from build123d import *

# Parameters (mm, degrees)
BOSS_EXTRUDE1_DEPTH     = 19.05
BOSS_EXTRUDE2_DEPTH     = 19.05
FILLET1_R               = 3.175
FILLET2_R               = 12.7
CUT_EXTRUDE1_DEPTH      = 957.630297054
CUT_EXTRUDE1_DEPTH_BACK = 957.630297054
SKETCH47_R              = 3.175
FILLET4_R               = 6.35
F_0_25_DIAMETER_HOLE1_D = 6.35
HOLE6_D                 = 3.175
HOLE6_DEPTH             = 38.1
HOLE6_CSINK_D           = 10.16
HOLE6_CSINK_ANGLE       = 82
HOLE6_TIP               = 0.953866233
HOLE9_D                 = 3.175
HOLE9_DEPTH             = 57.15
HOLE9_CSINK_D           = 10.16
HOLE9_CSINK_ANGLE       = 82
HOLE9_TIP               = 0.953866233
HOLE15_D                = 3.175
HOLE15_DEPTH            = 31.75
HOLE15_CSINK_D          = 10.16
HOLE15_CSINK_ANGLE      = 82
HOLE15_TIP              = 0.953866233


with BuildPart() as part:
    # Sketch1 → Boss-Extrude1 (new body)
    with BuildSketch(Plane.XY):
        Polygon((-247.274665566, 82.142339986), (-313.471036221, 60.427634584), (-546.587167873, 771.072405964), (-504.525442447, 784.870110692), (-417.251419261, 518.818903446), (-393.116774032, 526.735904121), align=None)
    extrude(amount=-BOSS_EXTRUDE1_DEPTH)

    # Sketch2 → Boss-Extrude2 (add, through all)
    with BuildSketch(Plane.XY):
        Polygon((-393.116774032, 526.735904121), (-336.901176267, 355.36500697), (-277.604402796, 374.816405204), (-281.415155825, 417.005352091), (-320.44916939, 493.083731154), (-290.280862854, 502.979981998), (-307.307307279, 554.884385267), align=None)
    extrude(amount=-BOSS_EXTRUDE2_DEPTH)

    # Fillet1
    fillet1_edges = [part.edges().sort_by_distance(p)[0] for p in [
        (-320.44916939, 493.083731154, -9.525),
    ]]
    fillet(fillet1_edges, radius=FILLET1_R)

    # Fillet2
    fillet2_edges = [part.edges().sort_by_distance(p)[0] for p in [
        (-336.901176267, 355.36500697, -9.525),
    ]]
    fillet(fillet2_edges, radius=FILLET2_R)

    # Sketch47 → Cut-Extrude1 (cut, two sides: drawn at the far end of the back side and taken through both)
    with BuildSketch(Plane(origin=(0, 0, -19.05), x_dir=(-1, 0, 0), z_dir=(0, 0, -1)).offset(-CUT_EXTRUDE1_DEPTH_BACK)):
        with Locations((417.251419261, 518.818903446)):
            Circle(SKETCH47_R)
    extrude(amount=CUT_EXTRUDE1_DEPTH + CUT_EXTRUDE1_DEPTH_BACK, mode=Mode.SUBTRACT)

    # Fillet4
    fillet4_edges = [part.edges().sort_by_distance(p)[0] for p in [
        (-418.241044345, 521.8357341, -9.525),
        (-414.234588607, 519.80852853, -9.525),
    ]]
    fillet(fillet4_edges, radius=FILLET4_R)

    # 0.25_ Diameter Hole1 (through all)
    with Locations(Plane.XY):
        with Locations((-563.45033927, 698.544682362), (-504.072834209, 517.534843147), (-343.557230523, 532.968767209), (-316.40575464, 541.875392969), (-305.317060721, 508.071973621), (-332.468536604, 499.165347862), (-384.427899865, 457.805801818), (-325.157897499, 477.248418201), (-305.715281117, 417.978415836), (-364.985283482, 398.535799453), (-323.698740376, 393.110483865), (-289.824308357, 404.222472403), (-287.772364418, 381.505347156), (-316.771364786, 371.99266929)):
            Hole(F_0_25_DIAMETER_HOLE1_D / 2)

    # Hole6
    with Locations(Plane(origin=(308.428945222, -359.406503987, -19.05), x_dir=(-0.9977564584489054, 0.06694811142592419, 0), z_dir=(0, 0, -1))):
        with Locations((615.24080496, 429.781381762), (710.914924699, 391.126528253), (904.68821492, 1078.38439498), (976.811864753, 1049.244548945), (835.937309391, 717.51890547), (711.83598555, 767.659094962)):
            CounterSinkHole(HOLE6_D / 2, HOLE6_CSINK_D / 2, depth=HOLE6_DEPTH, counter_sink_angle=HOLE6_CSINK_ANGLE)
            with Locations((0, 0, -(HOLE6_DEPTH + HOLE6_TIP / 2))):  # 118° drill point
                Cone(0, HOLE6_D / 2, HOLE6_TIP, mode=Mode.SUBTRACT)

    # Hole9
    with Locations(Plane(origin=(308.428945222, -359.406503987, -38.1), x_dir=(-0.9977564584489054, 0.06694811142592419, 0), z_dir=(0, 0, -1))):
        with Locations((848.944412528, 940.413642522), (885.927448463, 1031.949868564), (867.435930496, 986.181755543), (830.452894561, 894.645529501)):
            CounterSinkHole(HOLE9_D / 2, HOLE9_CSINK_D / 2, depth=HOLE9_DEPTH, counter_sink_angle=HOLE9_CSINK_ANGLE)
            with Locations((0, 0, -(HOLE9_DEPTH + HOLE9_TIP / 2))):  # 118° drill point
                Cone(0, HOLE9_D / 2, HOLE9_TIP, mode=Mode.SUBTRACT)

    # Hole15
    with Locations(Plane(origin=(-146.812587105, -508.741515314, 72.024999997), x_dir=(0, 0, 1), z_dir=(-0.9501828830204603, -0.3116929399504042, -1.2203303954814629e-15))):
        with Locations((-78.374999997, 1293.039195846), (-78.374999997, 1121.589195846), (78.374999997, 1121.589195846), (78.374999997, 1293.039195846)):
            CounterSinkHole(HOLE15_D / 2, HOLE15_CSINK_D / 2, depth=HOLE15_DEPTH, counter_sink_angle=HOLE15_CSINK_ANGLE)
            with Locations((0, 0, -(HOLE15_DEPTH + HOLE15_TIP / 2))):  # 118° drill point
                Cone(0, HOLE15_D / 2, HOLE15_TIP, mode=Mode.SUBTRACT)


solid = part.part
Could you check a few things on this model? Use its own coordinates, in mm. A direction names the side the tool comes from. Coordinates: 2 decimals unless noted, no trailing zeros. Loops run counter-clockwise (first coordinate to the right, second up) from the corner with the lowest first, then second, coordinate; pieces in that order, holes last. Notation, with made-up numbers: (56.5, -6.75) -> (76.5, -6.75) arc R17 cw to (76.5, 10.25) -> close; hole circle Ø1 at (36.5, 3.5). An arc over 180 degrees is marked (long way). Answer in a Markdown table with one row per item.
(1) Imagine slicing it at B-B (y = 429). List the corners of the cut face in (x, z) for me, plus the area to 3 significant figures.
Results found:
| item | result |
|---|---|
| outline | (-434.38, -19.05) -> (-287.57, -19.05) -> (-287.57, 0) -> (-434.38, 0) -> close |
| area | 2,800 mm^2 |
(2) Imagine slicing it at A-A (y = 666). List the corners of the cut face in (x, z) for me.
Results found:
| item | result |
|---|---|
| outline | (-512.12, -19.05) -> (-465.53, -19.05) -> (-465.53, 0) -> (-512.12, 0) -> close |
(3) Thinking about a two-plate mould opening in Y: for faces 3 (the face through (-375, 424, -19.05)), 4 (the face through (-525.851, 777.875, -9.392)), 5 (the face through (-299.82, 452.88, -9.39)), which applies, released by +Y, released by -Y, zero draft, split by the parting line, or undercut?
Results found:
| item | result |
|---|---|
| face 3 | zero draft |
| face 4 | released by +Y |
| face 5 | undercut |
(4) Will these pins go through, and if not, where does the flat tip stop? pin 1 Ø1.9 at (x, y) = (-506.42, 729.54) entering from +Z; pin 2 Ø8 at (x, z) = (-292.5, -13) entering from -Y; pin 3 Ø3 at (x, z) = (-287, -13) entering from -Y; pin 4 Ø1 at (y, z) = (217.5, -12.5) entering from -X.
Results found:
| item | result |
|---|---|
| pin 1 | passes through |
| pin 2 | stops at y = 65.99 |
| pin 3 | stops at y = 68.62 |
| pin 4 | stops at x = -365.16 |
(5) For faces 1 (the face through (-375, 398, 0)), 2 (the face through (-301.55, 366.96, -9.39)), which set-ups out of +Z, -Z, +X, -X, +Y, -Y let a thin tool reach every point of the face, with its end or its side?
Results found:
| item | result |
|---|---|
| face 1 | +Z, +X, -X, +Y, -Y |
| face 2 | +Z, -Z, +X |
(6) If I drill on probe 1 along X at (y, z) = (701.5, -2) (3 decimals); probe 2 along X at (y, z) = (460, -11); probe 3 along X at (y, z) = (206, -15.5), over which ranges is the centre line in solid material (lowest first)?
Results found:
| item | result |
|---|---|
| probe 1 | x = -523.765 to -477.177 |
| probe 2 | x = -444.54 to -386.72, -382.13 to -303.47 |
| probe 3 | x = -361.22 to -287.9 |
